Check sheet for the modelled part. Datum: model origin and axes. Units: mm. A direction names the side the tool comes from. Round coordinates to 2 decimals unless told otherwise and drop trailing zeros. Loops run counter-clockwise (first coordinate to the right, second up) from the corner with the lowest first, then second, coordinate; pieces in that order, holes last. Notation, with made-up numbers: M 29,87 L 80,87 A16 ccw 80,113 Z; hole C -16.5,-33.75 d5. An arc over 180 degrees is marked long. One line per question, with ' | ' between items. Start each with the question number.
(1) Thickness scan on probe 1 along Z at (x, y) = (0, 0.5); probe 2 along Z at (x, y) = (0, -7.35); probe 3 along X at (y, z) = (9.9, 0). Record the ranges inside material, lowest first. Write a range as [from, to].
(2) Tool access check on faces 1 (the face through (1, -5.2, -1)), 2 (the face through (-3, 10.3, -2)), 3 (the face through (-2.17, 10, -2.07)). Record the directions out of +Z, -Z, +X, -X, +Y, -Y that give a thin tool (end or side, any length) a straight path to the whole face; none if there is none.
(3) Section check A-A (y = 4.25). Record the boundary of the cut face in (x, z).
(4) Draft check along Z on faces 4 (the face through (1.08, 5.23, 4.88)), 5 (the face through (0.05, 5.42, 0.21)), 6 (the face through (-5, -10.3, 2)). Enter one of: +Z half, -Z half, draft (parallel to the pull), parting line (faces both ways), or undercut.
(5) Section check B-B (y = 8.5). Record the boundary of the cut face in (x, z).
(6) Go/stop test with flat-tipped pins: P1, Ø5, axis at x = 0, z = 0, coming from the +Y side; P2, Ø8, axis at y = -7, z = -4.5, coming from the -X side; P3, Ø3, axis at x = -2, z = 0, coming from the -Y side. Record where each tip stops, or that it passes through.
```python
from build123d import *

# Parameters (mm, degrees)
CUT_EXTRUDE_871_DEPTH  = 0.6
CHAMFER_1_SIZE         = 3
SKETCH_5_R             = 5.1
CUT_EXTRUDE_1040_DEPTH = 5.1
HOLE_WIZARD_M3_D       = 2.5
HOLE_WIZARD_M3_DEPTH   = 10
HOLE_WIZARD_M3_TIP     = 0.751075774


with BuildPart() as part:
    # Эскиз1 → Revolve 522 (revolve)
    with BuildSketch(Plane.XY):
        Polygon((0, 10.3), (-5, 10.3), (-5, 0.3), (-8, 0.3), (-8, -10.3), (0, -10.3), align=None)
    revolve(axis=Axis((0, 10.3, 0), (0, -1, 0)))

    # Эскиз4 → Cut-Extrude 871 (cut)
    with BuildSketch(Plane(origin=(0, 10.3, 0), x_dir=(1, 0, 0), z_dir=(0, 1, 0))):
        with BuildLine():
            Line((2.474108329, 1.696699141), (5.303300859, 1.696699141))
            Line((5.303300859, 1.696699141), (5.303300859, -5.303300859))
            Line((5.303300859, -5.303300859), (-1.696699141, -5.303300859))
            Line((-1.696699141, -5.303300859), (-1.696699141, -2.474108329))
            ThreePointArc((-1.696699141, -2.474108329), (-2.121320344, 2.121320344), (2.474108329, 1.696699141))
        make_face()
    extrude(amount=-CUT_EXTRUDE_871_DEPTH, mode=Mode.SUBTRACT)

    # Фаска1
    chamfer_1_edges = [part.edges().sort_by_distance(p)[0] for p in [
        (8, 0.3, 0),
    ]]
    chamfer(chamfer_1_edges, length=CHAMFER_1_SIZE - 0.0001)  # a hair under: the kernel refuses the full size

    # Эскиз5 → Cut-Extrude 1040 (cut)
    with BuildSketch(Plane.XZ.offset(10.3)):
        Circle(SKETCH_5_R)
    extrude(amount=-CUT_EXTRUDE_1040_DEPTH, mode=Mode.SUBTRACT)

    # Крепление магнита M3
    with Locations(Plane(origin=(0, -5.2, 0), x_dir=(-1, 0, 0), z_dir=(0, -1, 0))):
        with Locations((0, 0)):
            Hole(HOLE_WIZARD_M3_D / 2, depth=HOLE_WIZARD_M3_DEPTH)
            with Locations((0, 0, -(HOLE_WIZARD_M3_DEPTH + HOLE_WIZARD_M3_TIP / 2))):  # 118° drill point
                Cone(0, HOLE_WIZARD_M3_D / 2, HOLE_WIZARD_M3_TIP, mode=Mode.SUBTRACT)


solid = part.part
```
The answers:
1) probe 1: [-5, -1.25], [1.25, 5] | probe 2: [-8, -5.1], [5.1, 8] | probe 3: [-5, -3]
2) face 1: -Y | face 2: +Z, -Z, +X, -X, +Y | face 3: +Y
3) outline: C 0,0 d10; hole C 0,0 d2.5
4) face 4: parting line | face 5: undercut | face 6: draft
5) outline: C 0,0 d10
6) P1: y = 9.7 | P2: x = -7.98 | P3: y = -5.2
